from build123d import *

# Parameters (mm, degrees)
SKETCH_1_W          = 40
SKETCH_1_H          = 28.5
EXTRUDE_1_DEPTH     = 4
SKETCH_2_R          = 1.55
CUT_EXTRUDE_1_DEPTH = 25.880966621
SKETCH_3_R          = 1.55
CUT_EXTRUDE_2_DEPTH = 25.880966621
FILLET_1_R          = 3


with BuildPart() as part:
    # 草图1 → 凸台-拉伸1 (new body)
    with BuildSketch(Plane(origin=(0, 0, 0), x_dir=(1, 0, 0), z_dir=(0, 1, 0))):
        Rectangle(SKETCH_1_W, SKETCH_1_H)
        with BuildLine():
            Line((-14, 12.75), (14, 12.75))
            ThreePointArc((14, 12.75), (14.707106781, 12.457106781), (15, 11.75))
            Line((15, 11.75), (15, 9.75))
            ThreePointArc((15, 9.75), (14.707106781, 9.042893219), (14, 8.75))
            Line((14, 8.75), (-14, 8.75))
            ThreePointArc((-14, 8.75), (-14.707106781, 9.042893219), (-15, 9.75))
            Line((-15, 9.75), (-15, 11.75))
            ThreePointArc((-15, 11.75), (-14.707106781, 12.457106781), (-14, 12.75))
        make_face(mode=Mode.SUBTRACT)
    extrude(amount=EXTRUDE_1_DEPTH)

    # 草图2 → 切除-拉伸1 (cut, through all)
    with BuildSketch(Plane(origin=(0, 4, 0), x_dir=(1, 0, 0), z_dir=(0, 1, 0))):
        with Locations(Location((-15, -9.25, 0), (0, 0, 270))):
            Circle(SKETCH_2_R)
        with Locations(Location((5, -9.25, 0), (0, 0, 270))):
            Circle(SKETCH_2_R)
        with Locations(Location((15, -9.25, 0), (0, 0, 90))):
            Circle(SKETCH_2_R)
        with Locations(Location((-5, -9.25, 0), (0, 0, 90))):
            Circle(SKETCH_2_R)
    extrude(amount=-CUT_EXTRUDE_1_DEPTH, mode=Mode.SUBTRACT)

    # 草图3 → 切除-拉伸2 (cut, through all)
    with BuildSketch(Plane(origin=(0, 4, 0), x_dir=(1, 0, 0), z_dir=(0, 1, 0))):
        with Locations(Location((-15, -2.25, 0), (0, 0, 270))):
            Circle(SKETCH_3_R)
        with Locations(Location((-5, -2.25, 0), (0, 0, 270))):
            Circle(SKETCH_3_R)
        with Locations(Location((5, -2.25, 0), (0, 0, 270))):
            Circle(SKETCH_3_R)
        with Locations(Location((15, -2.25, 0), (0, 0, 270))):
            Circle(SKETCH_3_R)
    extrude(amount=-CUT_EXTRUDE_2_DEPTH, mode=Mode.SUBTRACT)

    # 圆角1
    fillet_1_edges = [part.edges().sort_by_distance(p)[0] for p in [
        (-20, 2, -14.25),
        (20, 2, -14.25),
    ]]
    fillet(fillet_1_edges, radius=FILLET_1_R)


solid = part.part
Can you work these out from the model? Positions are in its coordinate system, mm. A direction names the side the tool comes from. Coordinates: 2 decimals unless noted, no trailing zeros. Write each loop counter-clockwise with the first axis right and the second up, starting at its lowest first coordinate (ties: lowest second). Pieces come first, ordered by that corner, then holes. Notation, with made-up numbers: (55, 53) -> (60, 53) arc R28 cw to (60, 86) -> close; hole circle Ø4 at (55.25, 0.25). An arc over 180 degrees is marked (long way). Answer as CSV lines item,"result".
1) If I drill on line 1 (X direction, y = 2.8, z = 2.25); line 2 (Z direction, x = -8, y = 1.4); line 3 (X direction, y = 0.9, z = 10), over which ranges is the centre line in solid material (lowest first)? Write a range as from..to.
Check result:
line 1,"-20..-16.55, -13.45..-6.55, -3.45..3.45, 6.55..13.45, 16.55..20"
line 2,"-14.25..-12.75, -8.75..14.25"
line 3,"-20..-16.36, -13.64..-6.36, -3.64..3.64, 6.36..13.64, 16.36..20"
2) If we section it at B-B on z = 9.25: Please give me the cut outline in (x, y).
Check result:
outline,"(-20, 0) -> (-16.55, 0) -> (-16.55, 4) -> (-20, 4) -> close; (-13.45, 0) -> (-6.55, 0) -> (-6.55, 4) -> (-13.45, 4) -> close; (-3.45, 0) -> (3.45, 0) -> (3.45, 4) -> (-3.45, 4) -> close; (6.55, 0) -> (13.45, 0) -> (13.45, 4) -> (6.55, 4) -> close; (16.55, 0) -> (20, 0) -> (20, 4) -> (16.55, 4) -> close"
3) On a 3-axis mill with a long thin cutter (end or side, diameter ignored), from which of +Z, -Z, +X, -X, +Y, -Y can I reach the whole of each face in a straight line? I mean faces 1 (the flat face through (0, 2, -12.75)), 2 (the cylindrical face through (19.1, 2.03, -13.39)). Say none if no direction works.
Check result:
face 1,"+Y, -Y"
face 2,"-Z, +X, +Y, -Y"
4) If we section it at D-D on x = 5: Please give me the cut outline in (y, z), then the cut area to 3 significant figures.
Check result:
outline,"(0, -14.25) -> (4, -14.25) -> (4, -12.75) -> (0, -12.75) -> close; (0, -8.75) -> (4, -8.75) -> (4, 0.7) -> (0, 0.7) -> close; (0, 3.8) -> (4, 3.8) -> (4, 7.7) -> (0, 7.7) -> close; (0, 10.8) -> (4, 10.8) -> (4, 14.25) -> (0, 14.25) -> close"
area,"73.2 mm²"
5) Will these pins go through, and if not, where does the flat tip stop? P1, Ø1.5, axis at x = -15, z = 4, coming from the -Y side; P2, Ø1.9, axis at x = 5, z = 2.25, coming from the +Y side.
Check result:
P1,"y = 0"
P2,"through"
6) If we section it at C-C on y = 2.2: Count the separate pieces of the cut face and the enclosed holes in it, then the cut area to 3 significant figures.
Check result:
separate pieces,"1"
enclosed holes,"9"
area,"957 mm²"
7) If we section it at A-A on x = 12: Please give me the cut outline in (y, z), then the cut area to 3 significant figures.
Check result:
outline,"(0, -14.25) -> (4, -14.25) -> (4, -12.75) -> (0, -12.75) -> close; (0, -8.75) -> (4, -8.75) -> (4, 14.25) -> (0, 14.25) -> close"
area,"98.0 mm²"
8) If we mould it in two halves opening along X, with no side actions, what happens to faces 3 (the cylindrical face through (-13.463, 2.028, 2.048)), 4 (the cylindrical face through (-19.14, 2.03, -13.35)), 5 (the flat face through (0, 2, 14.25))? For each: +X half, -X half, draft (parallel to the pull), parting line (faces both ways), or undercut.
Check result:
face 3,"undercut"
face 4,"-X half"
face 5,"draft"
